```python
from build123d import *

# Parameters (mm, degrees)
F0_W      = 50
F0_H      = 50
F1_DEPTH  = 50
F2_R      = 6.25
F3_DEPTH  = 50.001
F4_R      = 6.25
F5_DEPTH  = 50.001
F6_R      = 6.25
F7_DEPTH  = 50.001
F8_W      = 15
F8_H      = 15
F9_DEPTH  = 50.001
F10_W     = 15
F10_H     = 15
F11_DEPTH = 50.001
F12_W     = 15
F12_H     = 15
F13_DEPTH = 50.001
F14_W     = 15
F14_H     = 15
F15_DEPTH = 50.001


with BuildPart() as f1:
    # F0 (on Top) → F1 (new body)
    with BuildSketch(Plane.XY):
        with Locations((-41.755149, -22.039188)):
            Rectangle(F0_W, F0_H)
    extrude(amount=F1_DEPTH)

    # F2 (on face) → F3 (cut, through all)
    with BuildSketch(Plane(origin=(-66.755149, 0, 0), x_dir=(0, -1, 0), z_dir=(-1, 0, 0))):
        with Locations((22.039188, 38.75)):
            Circle(F2_R)
    extrude(amount=-F3_DEPTH, mode=Mode.SUBTRACT)

    # F4 (on face) → F5 (cut, through all)
    with BuildSketch(Plane(origin=(-66.755149, 0, 0), x_dir=(0, -1, 0), z_dir=(-1, 0, 0))):
        with Locations((22.039188, 11.25)):
            Circle(F4_R)
    extrude(amount=-F5_DEPTH, mode=Mode.SUBTRACT)

    # F6 (on face) → F7 (cut, through all)
    with BuildSketch(Plane(origin=(0, 2.960812, 0), x_dir=(-1, 0, 0), z_dir=(0, 1, 0))):
        with Locations((41.755149, 25)):
            Circle(F6_R)
    extrude(amount=-F7_DEPTH, mode=Mode.SUBTRACT)

    # F8 (on face) → F9 (cut, through all)
    with BuildSketch(Plane.XY.offset(50)):
        with Locations((-59.255149, -39.539188)):
            Rectangle(F8_W, F8_H)
    extrude(amount=-F9_DEPTH, mode=Mode.SUBTRACT)

    # F10 (on face) → F11 (cut, through all)
    with BuildSketch(Plane.XY.offset(50)):
        with Locations((-59.255149, -4.539188)):
            Rectangle(F10_W, F10_H)
    extrude(amount=-F11_DEPTH, mode=Mode.SUBTRACT)

    # F12 (on face) → F13 (cut, through all)
    with BuildSketch(Plane.XY.offset(50)):
        with Locations((-24.255149, -4.539188)):
            Rectangle(F12_W, F12_H)
    extrude(amount=-F13_DEPTH, mode=Mode.SUBTRACT)

    # F14 (on face) → F15 (cut, through all)
    with BuildSketch(Plane.XY.offset(50)):
        with Locations((-24.255149, -39.539188)):
            Rectangle(F14_W, F14_H)
    extrude(amount=-F15_DEPTH, mode=Mode.SUBTRACT)


solid = f1.part
```
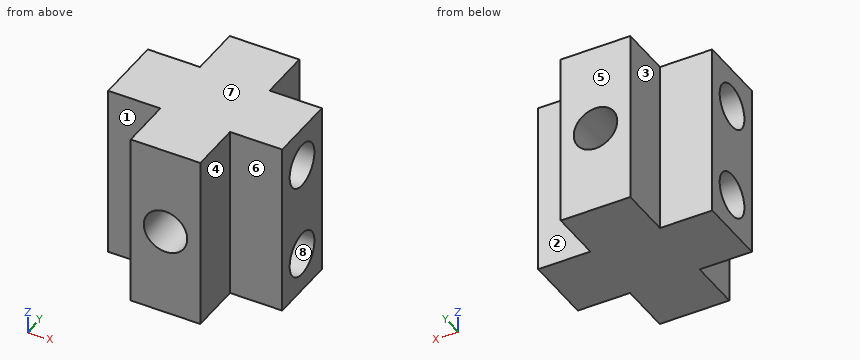
Could you check a few things on this model? Use its own coordinates, in mm. Face numbers are marked on the shaded views. A direction names the side the tool comes from. Round coordinates to 2 decimals unless told otherwise and drop trailing zeros. Loops run counter-clockwise (first coordinate to the right, second up) from the corner with the lowest first, then second, coordinate; pieces in that order, holes last. Notation, with made-up numbers: (72, 40) -> (120, 40) arc R17 cw to (120, 51) -> close; hole circle Ø3 at (71, 56.25). An arc over 180 degrees is marked (long way). One line per question, with ' | ' between items.
(1) If we section it at C-C on x = -19.5: List the corners of the cut face in (y, z) for me.
Model answer:
outline: (-32.04, 0) -> (-12.04, 0) -> (-12.04, 50) -> (-32.04, 50) -> close; hole circle Ø12.5 at (-22.04, 11.25); hole circle Ø12.5 at (-22.04, 38.75)
(2) Thinking about a two-plate mould opening in Y: for the marked faces 6, 7 and 8, which applies, released by +Y, released by -Y, zero draft, split by the parting line, or undercut?
Model answer:
face 6: released by -Y | face 7: zero draft | face 8: undercut
(3) For the marked faces 1, 2, 3, 4 and 5, which set-ups out of +Z, -Z, +X, -X, +Y, -Y let a thin tool reach every point of the face, with its end or its side?
Model answer:
face 1: +Z, -Z, -X, -Y | face 2: +Z, -Z, +X, +Y | face 3: +Z, -Z, -X, +Y | face 4: +Z, -Z, +X, -Y | face 5: +Z, -Z, +X, -X, +Y
(4) If we section it at D-D on z = 41: List the corners of the cut face in (x, y) for me.
Model answer:
outline: (-66.76, -32.04) -> (-51.76, -32.04) -> (-51.76, -47.04) -> (-31.76, -47.04) -> (-31.76, -32.04) -> (-16.76, -32.04) -> (-16.76, -27.87) -> (-66.76, -27.87) -> close; (-66.76, -16.21) -> (-16.76, -16.21) -> (-16.76, -12.04) -> (-31.76, -12.04) -> (-31.76, 2.96) -> (-51.76, 2.96) -> (-51.76, -12.04) -> (-66.76, -12.04) -> close
(5) For pin 1 Ø12 at (y, z) = (-3, 30) entering from -X; pin 2 Ø16.5 at (x, z) = (-22.5, 17) entering from -Y; pin 3 Ø7.5 at (y, z) = (-4.5, 33.5) entering from +X; pin 4 Ø11 at (x, z) = (-41.76, 25) entering from +Y, each with a flat end and sliding along its axis, tell me the tip position at first contact or that it passes through.
Model answer:
pin 1: stops at x = -51.76 | pin 2: stops at y = -32.04 | pin 3: stops at x = -31.76 | pin 4: passes through
(6) If I drill on probe 1 along Z at (x, y) = (-31.5, -26); probe 2 along Y at (x, z) = (-54, 11); probe 3 along Z at (x, y) = (-42, -27.5), over which ranges is the centre line in solid material (lowest first)?
Model answer:
probe 1: z = 0 to 6.42, 16.08 to 33.92, 43.58 to 50 | probe 2: y = -32.04 to -28.28, -15.79 to -12.04 | probe 3: z = 0 to 8.21, 14.29 to 18.75, 31.25 to 35.71, 41.79 to 50
(7) If we section it at A-A on z = 25: List the corners of the cut face in (x, y) for me, and give its area (3 significant figures).
Model answer:
outline: (-66.76, -32.04) -> (-51.76, -32.04) -> (-51.76, -47.04) -> (-48.01, -47.04) -> (-48.01, 2.96) -> (-51.76, 2.96) -> (-51.76, -12.04) -> (-66.76, -12.04) -> close; (-35.51, -47.04) -> (-31.76, -47.04) -> (-31.76, -32.04) -> (-16.76, -32.04) -> (-16.76, -12.04) -> (-31.76, -12.04) -> (-31.76, 2.96) -> (-35.51, 2.96) -> close | area: 975 mm^2
(8) If we section it at B-B on y = -13.5: List the corners of the cut face in (x, z) for me.
Model answer:
outline: (-66.76, 0) -> (-16.76, 0) -> (-16.76, 50) -> (-66.76, 50) -> close; hole circle Ø12.5 at (-41.76, 25)
